Can you work these out from the drawing? Everything is in mm from the part's minimum corner. A direction names the side the tool comes from. Round coordinates to 2 decimals unless told otherwise and drop trailing zeros. Loops run counter-clockwise (first coordinate to the right, second up) from the corner with the lowest first, then second, coordinate; pieces in that order, holes last. Notation, with made-up numbers: (48.25, 56) - (89.25, 56) arc R24 cw to (89.25, 82) - close; hole circle Ø10 at (33, 40.5). An arc over 180 degrees is marked (long way). Answer as CSV lines item,"result". Start each with the question number.
1) Which directions (+Z, -Z, +X, -X, +Y, -Y) give clear straight access to the entire face, cutting with the end or side of a thin tool? Please do the marked faces 1 and 2.
2) Suppose I cut it at B-B, the plane z = 7.5. Write out the boundary of the cut face in (x, y) (1 decimal).
3) I'm going to push flat-ended pins straight in: pin 1 Ø3 at (y, z) = (9, 9) entering from -X; pin 2 Ø2 at (y, z) = (2.5, 8) entering from -X; pin 3 Ø6 at (x, z) = (38.5, 6) entering from +Y; pin 4 Ø3 at (x, z) = (6.52, 6.52) entering from -Y. Where does each tip first touch, or does it pass through?
4) We'd pull the mould along Z, two halves only. Please class the marked faces 3, 4 and 5: pulls with the +Z half, pulls with the -Z half, needs draft (parallel to the pull), parting line crosses it, or undercut.
5) Please list where these lines run through material, in increasing order: line 1 along X through (y, z) = (1, 8.75) (1 decimal); line 2 along Y through (x, z) = (3, 5.75); line 3 along Z through (x, y) = (4.5, 4.75) (1 decimal).
6) Suppose I cut it at D-D, the plane x = 28.5. Write out the boundary of the cut face in (y, z) (1 decimal), then the cut area to 3 significant figures.
7) Suppose I cut it at A-A, the plane x = 43.5. Write out the boundary of the cut face in (y, z) (1 decimal).
8) Suppose I cut it at C-C, the plane y = 3.75. Write out the boundary of the cut face in (x, z).
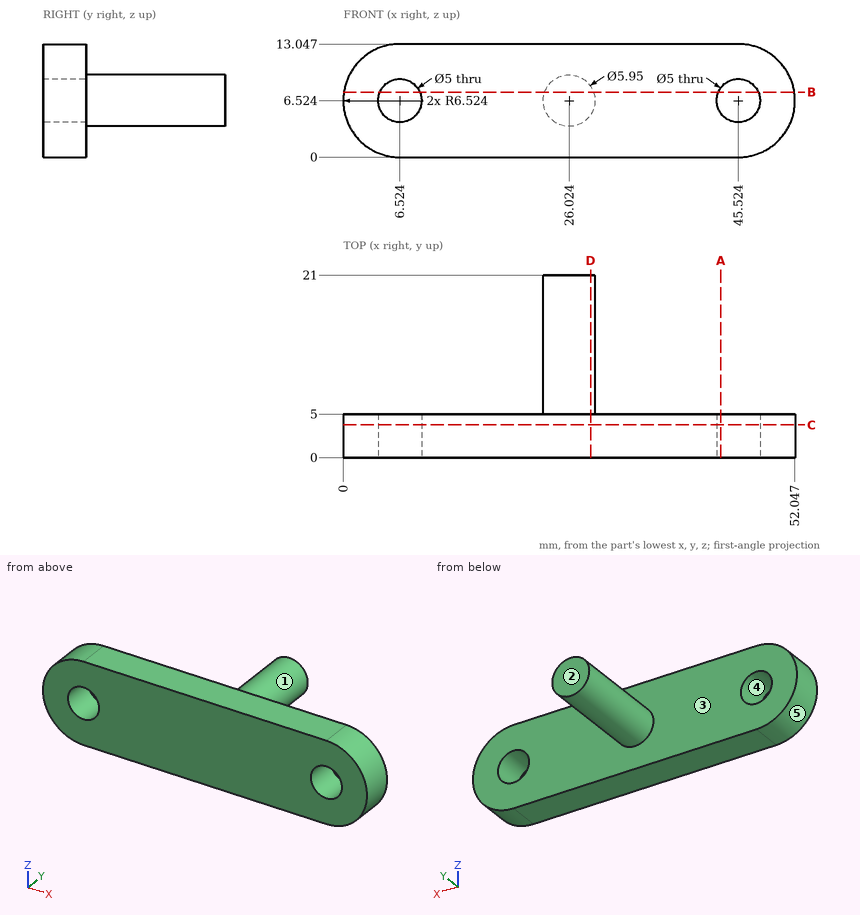
Filled sheet:
1,face 1,"+Y"
1,face 2,"+Z, -Z, +X, -X, +Y"
2,outline,"(0.1, 0) - (4.2, 0) - (4.2, 5) - (0.1, 5) - close; (8.8, 0) - (43.2, 0) - (43.2, 5) - (28.8, 5) - (28.8, 21) - (23.2, 21) - (23.2, 5) - (8.8, 5) - close; (47.8, 0) - (52, 0) - (52, 5) - (47.8, 5) - close"
3,pin 1,"x = 23.21"
3,pin 2,"x = 0.02"
3,pin 3,"y = 5"
3,pin 4,"through"
4,face 3,"needs draft"
4,face 4,"undercut"
4,face 5,"parting line crosses it"
5,line 1,"0.4 to 5.4, 7.7 to 44.4, 46.7 to 51.7"
5,line 2,"0 to 5"
5,line 3,"0.3 to 5.1, 8 to 12.7"
6,outline,"(0, 0) - (5, 0) - (5, 4.9) - (21, 4.9) - (21, 8.2) - (5, 8.2) - (5, 13) - (0, 13) - close"
6,area,"118 mm²"
7,outline,"(0, 0) - (5, 0) - (5, 5.1) - (0, 5.1) - close; (0, 8) - (5, 8) - (5, 13) - (0, 13) - close"
8,outline,"(6.52, 0) - (45.52, 0) arc R6.52 ccw to (45.52, 13.05) - (6.52, 13.05) arc R6.52 ccw to start; hole circle Ø5 at (6.52, 6.52); hole circle Ø5 at (45.52, 6.52)"
